Read the model definition and answer for the solid it produces. Units are mm, in the model's axes. Round coordinates to 2 decimals unless told otherwise and drop trailing zeros. Order: outer loops, then holes, each group sorted by start corner. A loop starts at its lowest first (then second) coordinate and runs counter-clockwise, first axis right, second up. Notation, with made-up numbers: (47.25, 72.5) -> (92.25, 72.5) arc R26 ccw to (92.25, 89.5) -> close; hole circle Ø8 at (-17.75, 35.25). An arc over 180 degrees is marked (long way). Use a Markdown table: item, result. Add a question column.
1. Section C-C, the plane y = -24 is taken. Give the vertices of the cut face in (x, z).
2. The mould has two halves that part along Y. Classify faces 1 (the face through (-100, 0, -3)), 2 (the face through (0.488, 21.804, -3.549)), 3 (the face through (-1, -30, -3)): +Y half, -Y half, draft (parallel to the pull), parting line (faces both ways), or undercut.
3. Consider L1, parallel to Y at x = 60, z = -4; L2, parallel to X at y = 0.5, z = -2; L3, parallel to Y at x = 61, z = -0.25. Determine where each line is inside the solid, lowest interval first. Write a range as [from, to].
4. Given pin 1 (3.5 mm diameter, centred on x = -60, y = -24, fed in from -Z), flat-ended and moving along its own axis, determine where the tip first touches the part or whether it passes through.
5. Section B-B, the plane x = 95 is taken. Give the vertices of the cut face in (y, z).
6. Section A-A, the plane y = 0 is taken. Give the vertices of the cut face in (x, z), then the cut area to 3 significant figures.
```python
from build123d import *

# Parameters (mm, degrees)
F0_W     = 200
F0_H     = 60
F1_DEPTH = 7
F2_D     = 4.5


with BuildPart() as f1:
    # F0 (on Top) → F1 (new body)
    with BuildSketch(Plane.XY):
        Rectangle(F0_W, F0_H)
    extrude(amount=-F1_DEPTH)

    # F2 (through all)
    with Locations(Plane.XY):
        with Locations((-60, 24), (60, 24), (60, -24), (-60, -24), (-95, 0), (95, 0), (0, 24), (0, -24)):
            Hole(F2_D / 2)


solid = f1.part
```
Verdict:
| question | item | result |
|---|---|---|
| 1 | outline | (-100, -7) -> (-62.25, -7) -> (-62.25, 0) -> (-100, 0) -> close; (-57.75, -7) -> (-2.25, -7) -> (-2.25, 0) -> (-57.75, 0) -> close; (2.25, -7) -> (57.75, -7) -> (57.75, 0) -> (2.25, 0) -> close; (62.25, -7) -> (100, -7) -> (100, 0) -> (62.25, 0) -> close |
| 2 | face 1 | draft |
| 2 | face 2 | undercut |
| 2 | face 3 | -Y half |
| 3 | L1 | y = [-30, -26.25], [-21.75, 21.75], [26.25, 30] |
| 3 | L2 | x = [-100, -97.19], [-92.81, 92.81], [97.19, 100] |
| 3 | L3 | y = [-30, -26.02], [-21.98, 21.98], [26.02, 30] |
| 4 | pin 1 | passes through |
| 5 | outline | (-30, -7) -> (-2.25, -7) -> (-2.25, 0) -> (-30, 0) -> close; (2.25, -7) -> (30, -7) -> (30, 0) -> (2.25, 0) -> close |
| 6 | outline | (-100, -7) -> (-97.25, -7) -> (-97.25, 0) -> (-100, 0) -> close; (-92.75, -7) -> (92.75, -7) -> (92.75, 0) -> (-92.75, 0) -> close; (97.25, -7) -> (100, -7) -> (100, 0) -> (97.25, 0) -> close |
| 6 | area | 1,340 mm2 |
